```python
from build123d import *

# Parameters (mm, degrees)
BOSS_EXTRUDE2_DEPTH = 20
SKETCH2_R           = 12.5
CUT_EXTRUDE1_DEPTH  = 80
SKETCH3_R           = 12.5
BOSS_EXTRUDE3_DEPTH = 10
SKETCH4_R           = 12.5
BOSS_EXTRUDE4_DEPTH = 10
CUT_EXTRUDE2_REACH  = 162
SKETCH5_R           = 5
SKETCH6_W           = 60
SKETCH6_H           = 20
CUT_EXTRUDE3_DEPTH  = 30


with BuildPart() as part:
    # Sketch1 → Boss-Extrude2 (new body)
    with BuildSketch(Plane.XY):
        Polygon((50, -115), (80, -115), (80, 115), (-80, 115), (-80, -115), (-50, -115), (-50, -15), (50, -15), align=None)
    extrude(amount=-BOSS_EXTRUDE2_DEPTH)

    # Sketch2 → Cut-Extrude1 (cut, symmetric)
    with BuildSketch(Plane(origin=(0, 0, 0), x_dir=(0, 0, -1), z_dir=(1, 0, 0))):
        with Locations((10, -122.5)):
            Circle(SKETCH2_R)
    extrude(amount=CUT_EXTRUDE1_DEPTH, both=True, mode=Mode.SUBTRACT)

    # Sketch3 → Boss-Extrude3 (add)
    with BuildSketch(Plane(origin=(80, 0, 0), x_dir=(0, 0, -1), z_dir=(1, 0, 0))):
        with Locations((10, -122.5)):
            Circle(SKETCH3_R)
    boss_extrude3 = extrude(amount=-BOSS_EXTRUDE3_DEPTH)

    # Mirror1: Boss-Extrude3 across plane
    add(boss_extrude3.mirror(Plane(origin=(0, 0, 0), x_dir=(0, 0, 1), z_dir=(1, 0, 0))))

    # Sketch4 → Boss-Extrude4 (add)
    with BuildSketch(Plane.ZY.offset(-50)):
        with Locations((-10, -122.5)):
            Circle(SKETCH4_R)
    boss_extrude4 = extrude(amount=-BOSS_EXTRUDE4_DEPTH)

    # Mirror2: Boss-Extrude4 across plane
    add(boss_extrude4.mirror(Plane(origin=(0, 0, 0), x_dir=(0, 0, 1), z_dir=(1, 0, 0))))

    # Sketch5 → Cut-Extrude2 (cut, up to next)
    with BuildSketch(Plane(origin=(80, 0, 0), x_dir=(0, 0, -1), z_dir=(1, 0, 0)), mode=Mode.PRIVATE) as cut_extrude2_sk1:
        with Locations((10, 100)):
            Circle(SKETCH5_R)
    cut_extrude2_tool1 = extrude(cut_extrude2_sk1.sketch, amount=-CUT_EXTRUDE2_REACH, mode=Mode.PRIVATE) & part.part
    add(cut_extrude2_tool1.solids().sort_by_distance((80, 100, -10))[0], mode=Mode.SUBTRACT)

    # Sketch6 → Cut-Extrude3 (cut)
    with BuildSketch(Plane(origin=(0, 115, 0), x_dir=(1, 0, 0), z_dir=(0, 1, 0))):
        with Locations((0, 10)):
            Rectangle(SKETCH6_W, SKETCH6_H)
    extrude(amount=-CUT_EXTRUDE3_DEPTH, mode=Mode.SUBTRACT)


solid = part.part
```
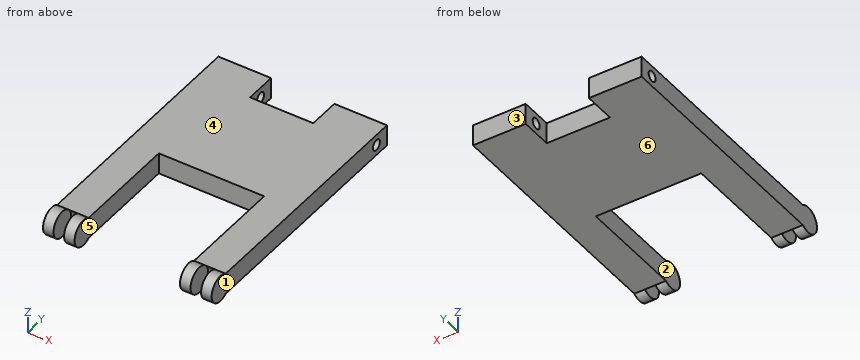
For this review, take the finished solid that the model builds, in its own axes (mm). Face numbers are marked on the shaded views. A direction names the side the tool comes from. Give positions to 0.01 mm unless a question says otherwise; leave off trailing zeros. Order: outer loops, then holes, each group sorted by start corner. A loop starts at its lowest first (then second) coordinate and runs counter-clockwise, first axis right, second up.
1) Insertion check: pin 1 (1.5 mm diameter, centred on x = -16.5, z = -13.5, fed in from -Y); pin 2 (5 mm diameter, centred on x = 24, z = -0.5, fed in from +Y); pin 3 (12 mm diameter, centred on x = -28, y = 16.5, fed in from -Z). Each pin has a flat end and moves straight along its axis. Give the tip position at first contact, or say it passes through.
2) Wall thickness on line 1 (Y direction, x = -42.5, z = -10); line 2 (Y direction, x = 69, z = -10); line 3 (X direction, y = -81, z = -15.5): over which ranges is each line inside the solid? List them lowest first.
3) Take a section at A-A (y = 100). Give the boundary of the cut face in (x, z).
4) The part is to be moulded in two halves that separate along X. For the marked faces 1, 2 and 3, say which applies: released by +X, released by -X, zero draft, split by the parting line, or undercut.
5) Take a section at D-D (x = 10). Give the boundary of the cut face in (y, z), then the cut area to 3 significant figures.
6) Take a section at B-B (z = -10). Give the boundary of the cut face in (x, y), then the cut area to 3 significant figures.
7) For the marked faces 4, 5 and 6, list the 3-axis set-ups (+Z, -Z, +X, -X, +Y, -Y) from which the entire face can be reached by the end or side of a thin tool; tool diameter is ignored.
8) Take a section at C-C (x = 53). Give the boundary of the cut face in (y, z).
Derived:
1. pin 1: stops at y = -15
1. pin 2: stops at y = 85
1. pin 3: stops at z = -20
2. line 1: y = -15 to 95, 105 to 115
2. line 2: y = -110 to 95, 105 to 115
2. line 3: x = -80 to -50, 50 to 80
3. outline: (-80, -20) - (-30, -20) - (-30, -15) - (-80, -15) - close; (-80, -5) - (-30, -5) - (-30, 0) - (-80, 0) - close; (30, -20) - (80, -20) - (80, -15) - (30, -15) - close; (30, -5) - (80, -5) - (80, 0) - (30, 0) - close
4. face 1: released by +X
4. face 2: undercut
4. face 3: zero draft
5. outline: (-15, -20) - (85, -20) - (85, 0) - (-15, 0) - close
5. area: 2,000 mm2
6. outline: (-80, -135) - (-70, -135) - (-70, -110) - (-60, -110) - (-60, -135) - (-50, -135) - (-50, -15) - (50, -15) - (50, -135) - (60, -135) - (60, -110) - (70, -110) - (70, -135) - (80, -135) - (80, 95) - (30, 95) - (30, 85) - (-30, 85) - (-30, 95) - (-80, 95) - close; (-80, 105) - (-30, 105) - (-30, 115) - (-80, 115) - close; (30, 105) - (80, 105) - (80, 115) - (30, 115) - close
6. area: 24,700 mm2
7. face 4: +Z, +X, -X, +Y
7. face 5: +Z, -Z, -Y
7. face 6: -Z, +X, -X, +Y
8. outline: (-115, -20) - (115, -20) - (115, 0) - (-115, 0) arc R12.5 ccw (long way) to start; hole circle Ø10 at (100, -10)
